Could you check a few things on this model? Use its own coordinates, in mm. Give positions to 0.01 mm unless a question says otherwise; leave off trailing zeros. Order: outer loops, then holes, each group sorted by start corner. A loop starts at its lowest first (then second) coordinate and runs counter-clockwise, first axis right, second up.
Autodesk Inventor part; units mm, degrees
ref_plane "Work Plane1" through (1104.5696, 91.5553, 211.8164) normal (0, 1, 0) x (-1, 0, 0)
ref_plane "YZ Plane" through (0, 0, 0) normal (1, 0, 0) x (0, 1, 0)
ref_plane "XZ Plane" through (0, 0, 0) normal (0, 1, 0) x (-1, 0, 0)
ref_plane "Work Plane1" through (1104.5696, 91.5553, 211.8164) normal (0, 1, 0) x (-1, 0, 0)
sketch "Sketch1" plane through (1104.5696, 91.5553, 211.8164) normal (0, 1, 0) x (-1, 0, 0)
  arc A0 (57.6551, 1254.9955) -> (57.6551, 1150.0245) centre (104.395, 1202.51) ccw
  line L0 (-26.3951, 1291) -> (133.6049, 1291)
  line L1 (133.6049, 1019) -> (-26.3951, 1019)
  line L2 (-26.3951, 1249) -> (-26.3951, 1291)
  line L3 (179.6049, 2285) -> (179.6049, 25)
  line L4 (179.6049, 1019) -> (179.6049, 1291.0001)
  line L5 (-72.3951, 25) -> (-72.3951, 2285)
  line L6 (179.6049, 1291.0001) -> (-222.3951, 1291.0001)
  line L7 (179.6049, 1019) -> (-222.3951, 1019)
  line L8 (-222.3951, 25) -> (-222.3951, 2285)
  line L9 (-222.3951, 1291.0001) -> (-222.3951, 1019)
  point P0 (1104.5696, -211.8164)
  point P1 (-72.3951, 1291.0001)
  point P2 (-72.3951, 1019)
  point P3 (154, 1291)
  point P4 (4, 1291)
extrude "Extrusion1" add sketch "Sketch1" along normal blind 12.7
sketch "Sketch2" plane through (1104.5696, 104.2553, 211.8164) normal (0, 1, 0) x (1, 0, 0)
  line L0 (222.3951, -1019) -> (-179.6049, -1019) construction
  line L1 (-179.6049, -1019) -> (-179.6049, -1291.0001) construction
  line L2 (-179.6049, -1291.0001) -> (222.3951, -1291.0001) construction
  line L3 (222.3951, -1291.0001) -> (222.3951, -1019) construction
  line L4 (-179.6049, -1291.0001) -> (222.3951, -1291.0001) construction
  line L5 (21.3951, -1291.0001) -> (21.3951, -1019) construction
  line L6 (-179.6049, -1019) -> (-179.6049, -1291.0001) construction
  line L7 (-179.6049, -1155) -> (222.3951, -1155) construction
  point P0 (-1104.5696, 211.8164)
  point P1 (-159.6049, -1266.0001)
  point P2 (50.3951, -1266.0001)
  point P3 (-159.6049, -1044)
  point P4 (50.3951, -1044)
  dimension "d16" = 25
  dimension "d17" = 20
  dimension "d18" = 25
  dimension "d19" = 210
hole "Hole1" at (944.9647, 104.2553, 1477.8164) at (944.9647, 104.2553, 1255.8164) at (1154.9647, 104.2553, 1255.8164) at (1154.9647, 104.2553, 1477.8164) direction (0, -1, 0) diameter 12 end through all
fillet "Fillet1" radius 100 1 edges at (1326.9647, 97.9053, 1502.8164)
fillet "Fillet2" radius 100 1 edges at (1326.9647, 97.9053, 1230.8164)
sketch "Sketch3" plane through (1104.5696, 104.2553, 211.8164) normal (0, 1, 0) x (1, 0, 0)
  line L0 (-129.6049, -1110.5) -> (-40.6049, -1110.5)
  line L1 (-40.6049, -1110.5) -> (-40.6049, -1199.5)
  line L2 (-40.6049, -1199.5) -> (-129.6049, -1199.5)
  line L3 (-129.6049, -1199.5) -> (-129.6049, -1110.5)
  line L4 (-179.6049, -1019) -> (-179.6049, -1291.0001)
  line L5 (-179.6049, -1155) -> (-143.519, -1155)
  point P0 (-1104.5696, 211.8164)
  dimension "d20" = 89
  dimension "d21" = 89
  dimension "d22" = 50
hole "Hole2" at (974.9647, 104.2553, 1322.3164) at (1063.9647, 104.2553, 1322.3164) at (1063.9647, 104.2553, 1411.3164) at (974.9647, 104.2553, 1411.3164) direction (0, -1, 0) diameter 10 end through all
properties part number "PlacaInferior" material "Steel ASTM A36"
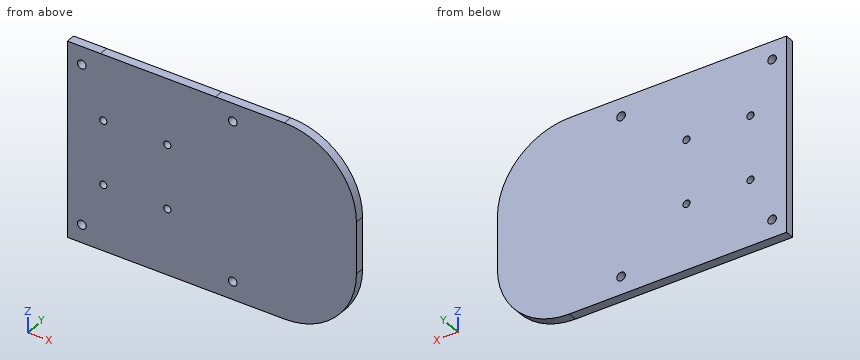
Item 1: Imagine slicing it at C-C on z = 1446.5. List the corners of the cut face in (x, y) for me.
Findings:
outline: (924.96, 91.56) - (1316.92, 91.56) - (1316.92, 104.26) - (924.96, 104.26) - close
Item 2: Imagine slicing it at B-B on x = 1270.5. List the corners of the cut face in (y, z) for me.
Findings:
outline: (91.56, 1240.79) - (104.26, 1240.79) - (104.26, 1492.84) - (91.56, 1492.84) - close
Item 3: Imagine slicing it at A-A on y = 94.5. Give the number of separate pieces and of enclosed holes in the cut face, then the cut area to 3 significant figures.
Findings:
separate pieces: 1
enclosed holes: 8
area: 104,000 mm2
Item 4: For pin 1 (5 mm diameter, centred on y = 95.5, z = 1294, fed in from +X), with a flat end and sliding along its axis, tell me the tip position at first contact or that it passes through.
Findings:
pin 1: stops at x = 1320.89
Item 5: Please list where these lines run through material, in increasing order: line 1 along X through (y, z) = (95.25, 1412); line 2 along X through (y, z) = (95.5, 1413.5); line 3 along X through (y, z) = (102, 1491).
Findings:
line 1: x = 924.96 to 970.01, 979.92 to 1059.01, 1068.92 to 1326.54
line 2: x = 924.96 to 970.47, 979.46 to 1059.47, 1068.46 to 1326.39
line 3: x = 924.96 to 1274.12
